```python
from build123d import *

# Parameters (mm, degrees)
IZIM1_R                     = 1.875
IZIM1_R_2                   = 2
Y_KSEKLIK_EKSTR_ZYON2_DEPTH = 3
KES_EKSTR_ZYON1_DEPTH       = 2.4
IZIM3_R                     = 3.3
IZIM3_R_2                   = 1.875
Y_KSEKLIK_EKSTR_ZYON3_DEPTH = 3


with BuildPart() as part:
    # Çizim1 → Yükseklik-Ekstrüzyon2 (new body)
    with BuildSketch(Plane.XY):
        with BuildLine():
            Line((-50, 45), (50, 45))
            ThreePointArc((50, 45), (57.071067812, 42.071067812), (60, 35))
            Line((60, 35), (60, -35))
            ThreePointArc((60, -35), (57.071067812, -42.071067812), (50, -45))
            Line((50, -45), (-50, -45))
            ThreePointArc((-50, -45), (-57.071067812, -42.071067812), (-60, -35))
            Line((-60, -35), (-60, 35))
            ThreePointArc((-60, 35), (-57.071067812, 42.071067812), (-50, 45))
        make_face()
        with Locations((-50.925, 38.05)):
            Circle(IZIM1_R, mode=Mode.SUBTRACT)
        with Locations((50.925, 38.05)):
            Circle(IZIM1_R, mode=Mode.SUBTRACT)
        with Locations((-50.925, -38.05)):
            Circle(IZIM1_R, mode=Mode.SUBTRACT)
        with Locations((50.925, -38.05)):
            Circle(IZIM1_R, mode=Mode.SUBTRACT)
        with Locations((-38.075, -13.95)):
            Circle(IZIM1_R_2, mode=Mode.SUBTRACT)
        with BuildLine():
            Line((-31.075, -38.05), (31.075, -38.05))
            ThreePointArc((31.075, -38.05), (33.196320344, -37.171320344), (34.075, -35.05))
            Line((34.075, -35.05), (34.075, -20.95))
            ThreePointArc((34.075, -20.95), (33.196320344, -18.828679656), (31.075, -17.95))
            Line((31.075, -17.95), (-31.075, -17.95))
            ThreePointArc((-31.075, -17.95), (-33.196320344, -18.828679656), (-34.075, -20.95))
            Line((-34.075, -20.95), (-34.075, -35.05))
            ThreePointArc((-34.075, -35.05), (-33.196320344, -37.171320344), (-31.075, -38.05))
        make_face(mode=Mode.SUBTRACT)
        with BuildLine():
            Line((50.925, 28.05), (50.925, -6.95))
            ThreePointArc((50.925, -6.95), (50.046320344, -9.071320344), (47.925, -9.95))
            Line((47.925, -9.95), (43.925, -9.95))
            ThreePointArc((43.925, -9.95), (41.803679656, -9.071320344), (40.925, -6.95))
            Line((40.925, -6.95), (40.925, 38.05))
            ThreePointArc((40.925, 38.05), (47.996067812, 35.121067812), (50.925, 28.05))
        make_face(mode=Mode.SUBTRACT)
        with BuildLine():
            Line((-31.075, 38.05), (31.075, 38.05))
            ThreePointArc((31.075, 38.05), (33.196320344, 37.171320344), (34.075, 35.05))
            Line((34.075, 35.05), (34.075, -6.95))
            ThreePointArc((34.075, -6.95), (33.196320344, -9.071320344), (31.075, -9.95))
            Line((31.075, -9.95), (-31.075, -9.95))
            ThreePointArc((-31.075, -9.95), (-33.196320344, -9.071320344), (-34.075, -6.95))
            Line((-34.075, -6.95), (-34.075, 35.05))
            ThreePointArc((-34.075, 35.05), (-33.196320344, 37.171320344), (-31.075, 38.05))
        make_face(mode=Mode.SUBTRACT)
        with BuildLine():
            Line((-50.925, 28.05), (-50.925, -6.95))
            ThreePointArc((-50.925, -6.95), (-50.046320344, -9.071320344), (-47.925, -9.95))
            Line((-47.925, -9.95), (-43.925, -9.95))
            ThreePointArc((-43.925, -9.95), (-41.803679656, -9.071320344), (-40.925, -6.95))
            Line((-40.925, -6.95), (-40.925, 38.05))
            ThreePointArc((-40.925, 38.05), (-47.996067812, 35.121067812), (-50.925, 28.05))
        make_face(mode=Mode.SUBTRACT)
        with BuildLine():
            Line((-47.925, -17.95), (-43.925, -17.95))
            ThreePointArc((-43.925, -17.95), (-41.803679656, -18.828679656), (-40.925, -20.95))
            Line((-40.925, -20.95), (-40.925, -38.05))
            ThreePointArc((-40.925, -38.05), (-47.996067812, -35.121067812), (-50.925, -28.05))
            Line((-50.925, -28.05), (-50.925, -20.95))
            ThreePointArc((-50.925, -20.95), (-50.046320344, -18.828679656), (-47.925, -17.95))
        make_face(mode=Mode.SUBTRACT)
        with BuildLine():
            Line((50.925, -20.95), (50.925, -28.05))
            ThreePointArc((50.925, -28.05), (47.996067812, -35.121067812), (40.925, -38.05))
            Line((40.925, -38.05), (40.925, -20.95))
            ThreePointArc((40.925, -20.95), (41.803679656, -18.828679656), (43.925, -17.95))
            Line((43.925, -17.95), (47.925, -17.95))
            ThreePointArc((47.925, -17.95), (50.046320344, -18.828679656), (50.925, -20.95))
        make_face(mode=Mode.SUBTRACT)
    extrude(amount=Y_KSEKLIK_EKSTR_ZYON2_DEPTH)

    # Çizim2 → Kes-Ekstrüzyon1 (cut)
    with BuildSketch(Plane(origin=(0, 0, 0), x_dir=(-1, 0, 0), z_dir=(0, 0, -1))):
        Polygon((-53.35905554, -36.010709201), (-53.908105407, -39.138308533), (-51.474049867, -41.177599331), (-48.49094446, -40.089290799), (-47.941894593, -36.961691467), (-50.375950133, -34.922400669), align=None)
        Polygon((48.49094446, -36.010709201), (47.941894593, -39.138308533), (50.375950133, -41.177599331), (53.35905554, -40.089290799), (53.908105407, -36.961691467), (51.474049867, -34.922400669), align=None)
        Polygon((48.49094446, 40.089290799), (47.941894593, 36.961691467), (50.375950133, 34.922400669), (53.35905554, 36.010709201), (53.908105407, 39.138308533), (51.474049867, 41.177599331), align=None)
        Polygon((-53.35905554, 40.089290799), (-53.908105407, 36.961691467), (-51.474049867, 34.922400669), (-48.49094446, 36.010709201), (-47.941894593, 39.138308533), (-50.375950133, 41.177599331), align=None)
    extrude(amount=-KES_EKSTR_ZYON1_DEPTH, mode=Mode.SUBTRACT)

    # Çizim3 → Yükseklik-Ekstrüzyon3 (add)
    # profile 1 of 4: a face of its own
    with BuildSketch(Plane.XY.offset(3)):
        with Locations((-50.925, 38.05)):
            Circle(IZIM3_R)
        with Locations(Location((-50.925, 38.05, 0), (0, 0, 180))):
            Circle(IZIM3_R_2, mode=Mode.SUBTRACT)
    # profile 2 of 4: a face of its own
    with BuildSketch(Plane.XY.offset(3)):
        with Locations((50.925, 38.05)):
            Circle(IZIM3_R)
        with Locations(Location((50.925, 38.05, 0), (0, 0, 180))):
            Circle(IZIM3_R_2, mode=Mode.SUBTRACT)
    # profile 3 of 4: a face of its own
    with BuildSketch(Plane.XY.offset(3)):
        with Locations((-50.925, -38.05)):
            Circle(IZIM3_R)
        with Locations(Location((-50.925, -38.05, 0), (0, 0, 180))):
            Circle(IZIM3_R_2, mode=Mode.SUBTRACT)
    # profile 4 of 4: a face of its own
    with BuildSketch(Plane.XY.offset(3)):
        with Locations((50.925, -38.05)):
            Circle(IZIM3_R)
        with Locations(Location((50.925, -38.05, 0), (0, 0, 180))):
            Circle(IZIM3_R_2, mode=Mode.SUBTRACT)
    extrude(amount=Y_KSEKLIK_EKSTR_ZYON3_DEPTH)


solid = part.part
```
The model under review builds one solid part; all positions refer to its coordinate system, in mm. A direction names the side the tool comes from. Round coordinates to 2 decimals unless told otherwise and drop trailing zeros. Write each loop counter-clockwise with the first axis right and the second up, starting at its lowest first coordinate (ties: lowest second). Pieces come first, ordered by that corner, then holes. Notation, with made-up numbers: (55.5, 22) - (71.5, 22) arc R22 ccw to (71.5, 45) - close; hole circle Ø11 at (77, -31). An arc over 180 degrees is marked (long way). One line per question, with ' | ' between items.
Item 1: Add section D-D, the plane y = 31. Give the boundary of the cut face in (x, z) (3 decimals), then the cut area to 3 significant figures.
Resolved:
outline: (-60, 0) - (-50.48, 0) - (-50.48, 3) - (-60, 3) - close; (-40.925, 0) - (-34.075, 0) - (-34.075, 3) - (-40.925, 3) - close; (34.075, 0) - (40.925, 0) - (40.925, 3) - (34.075, 3) - close; (50.48, 0) - (60, 0) - (60, 3) - (50.48, 3) - close | area: 98.2 mm2
Item 2: Add section B-B, the plane y = -13.95. Give the boundary of the cut face in (x, z) (3 decimals), then the cut area to 3 significant figures.
Resolved:
outline: (-60, 0) - (-40.075, 0) - (-40.075, 3) - (-60, 3) - close; (-36.075, 0) - (60, 0) - (60, 3) - (-36.075, 3) - close | area: 348 mm2
Item 3: Add section C-C, the plane z = 1.2. State how many separate pieces and enclosed holes the cut face has, then the cut area to 3 significant figures.
Resolved:
separate pieces: 1 | enclosed holes: 11 | area: 4,710 mm2
Item 4: The part is to be moulded in two halves that separate along Y. For faces 4 (the face through (50, -40.64, 1.18)), 5 (the face through (1, 41, 0)), say which applies: pulls with the +Y half, pulls with the -Y half, needs draft (parallel to the pull), parting line crosses it, or undercut.
Resolved:
face 4: undercut | face 5: needs draft
Item 5: Add section A-A, the plane x = -18. Give the boundary of the cut face in (y, z), then the cut area to 3 significant figures.
Resolved:
outline: (-45, 0) - (-38.05, 0) - (-38.05, 3) - (-45, 3) - close; (-17.95, 0) - (-9.95, 0) - (-9.95, 3) - (-17.95, 3) - close; (38.05, 0) - (45, 0) - (45, 3) - (38.05, 3) - close | area: 65.7 mm2
Item 6: For P1, Ø3.5, axis at x = 50.925, y = -38.05, coming from the -Z side, flat-tipped, find the tip position at first contact; note if it passes through.
Resolved:
P1: passes through
Item 7: For faces 1 (the face through (60, 0, 1)), 2 (the face through (-34.075, 14, 1)), 3 (the face through (49.14, 40.14, 1.18)), list the 3-axis set-ups (+Z, -Z, +X, -X, +Y, -Y) from which the entire face can be reached by the end or side of a thin tool; tool diameter is ignored.
Resolved:
face 1: +Z, -Z, +X, +Y, -Y | face 2: +Z, -Z | face 3: -Z
Item 8: To check wall thickness, follow probe 1 along X at (y, z) = (-25, 0.55) (3 decimals); probe 2 along Y at (x, z) = (-21, 2.95); probe 3 along Y at (x, z) = (47.5, 2.05). State the ranges of each line that lie inside material, in increasing order.
Resolved:
probe 1: x = -60 to -50.925, -40.925 to -34.075, 34.075 to 40.925, 50.925 to 60 | probe 2: y = -45 to -38.05, -17.95 to -9.95, 38.05 to 45 | probe 3: y = -45 to -35.58, -17.95 to -9.95, 35.58 to 45
